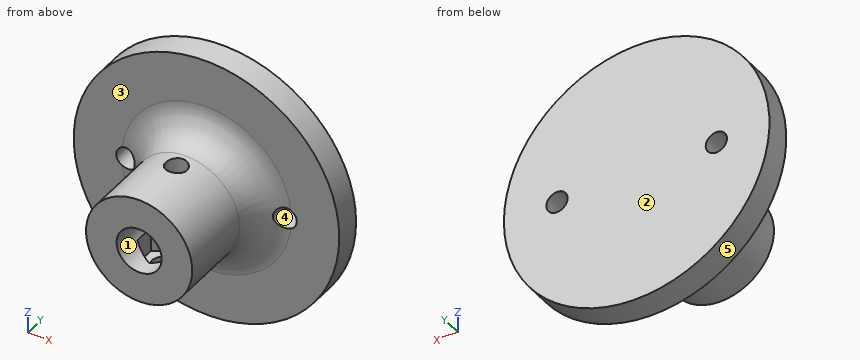
Solid Edge part; units mm, degrees
sketch "Sketch1" plane through (0, 0, 0) normal (0, -1, 0) x (1, 0, 0)
  circle A0 centre (0, 0) radius 10
  circle A1 centre (0, 0) radius 4.25
extrude "Protrusion1" add sketch "Sketch1" along normal blind 20
sketch "Sketch2" plane through (0, 0, 0) normal (0, -1, 0) x (1, 0, 0)
  circle A0 centre (-15, 0) radius 2
  circle A1 centre (0, 0) radius 25
  circle A2 centre (15, 0) radius 2
extrude "ExtrudedProtrusion_3" add sketch "Sketch2" against normal blind 5
fillet "Round_2" radius 6 1 edges at (-10, 0, 0)
sketch "Sketch3" plane through (0, 0, 0) normal (0, 0, 1) x (1, 0, 0)
  line L0 (-3.5, -10.9793) -> (-3.5, -15.0207)
  line L1 (-3.5, -15.0207) -> (0, -17.0415)
  line L2 (0, -17.0415) -> (3.5, -15.0207)
  line L3 (3.5, -15.0207) -> (3.5, -10.9793)
  line L4 (3.5, -10.9793) -> (0, -8.9585)
  line L5 (0, -8.9585) -> (-3.5, -10.9793)
extrude "ExtrudedCutout_3" cut sketch "Sketch3" against normal blind 7
sketch "Sketch4" plane through (0, 0, 0) normal (0, 0, 1) x (1, 0, 0)
  line L0 (0, -13) -> (3.5, -10.9793)
  line L1 (3.5, -10.9793) -> (3.5, -6.9378)
  line L2 (3.5, -6.9378) -> (0, -4.9171)
  line L3 (0, -4.9171) -> (-3.5, -6.9378)
  line L4 (-3.5, -6.9378) -> (-3.5, -10.9793)
  line L5 (-3.5, -10.9793) -> (0, -13)
extrude "ExtrudedCutout_4" cut sketch "Sketch4" along normal blind 7
sketch "Sketch5" plane through (0, 0, -11) normal (0, 0, 1) x (1, 0, 0)
  circle A0 centre (0, -13) radius 2
extrude "ExtrudedCutout_5" cut sketch "Sketch5" along normal blind 8
sketch "Sketch6" plane through (0, 0, 11) normal (0, 0, 1) x (1, 0, 0)
  circle A0 centre (0, -8.9585) radius 2
extrude "ExtrudedCutout_6" cut sketch "Sketch6" against normal blind 8
Source: CAD feature listing. Evaluate the final solid. Frame: model axes, mm. Face numbers are marked on the shaded views. A direction names the side the tool comes from. Round coordinates to 2 decimals unless told otherwise and drop trailing zeros. Loops run counter-clockwise (first coordinate to the right, second up) from the corner with the lowest first, then second, coordinate; pieces in that order, holes last. Notation, with made-up numbers: M -2.75,80.5 L 3.25,80.5 A8 ccw 3.25,85.5 Z; hole C 50.5,80.5 d1. An arc over 180 degrees is marked long. Use a Markdown table: item, result. Add a question column.
1. Line query: line 1 (X direction, y = -13, z = -9.05); line 2 (Z direction, x = 0, y = -16); line 3 (Z direction, x = 0, y = -10.5). Output: solid intervals per line, ascending.
2. Section query A-A on z = 0. Return the cut outline in (x, y).
3. Reachability of the marked faces 1 and 2 from +Z, -Z, +X, -X, +Y, -Y: full face, straight path, thin tool, end or side. Return the list, or none.
4. Section query B-B on y = 3.25. Return the cut outline in (x, z).
5. Section query D-D on z = 18. Return the cut outline in (x, y), then the cut area to 3 significant figures.
6. Contact query for flat-ended pins moving along their axis: P1, Ø4.5, axis at y = -13.5, z = -5.5, coming from the +X side; P2, Ø2, axis at x = 1.5, y = -9.5, coming from the -Z side; P3, Ø2.5, axis at x = 15, z = 0, coming from the -Y side; P4, Ø7.5, axis at x = 0.5, y = -11.5, coming from the +Z side. Output: stop coordinate, or through.
7. Section query C-C on y = -2.25. Return the cut outline in (x, z), then the cut area to 3 significant figures.
8. Mould query, pull axis X, two halves, no side actions, for the marked faces 3, 4 and 5. Classes: pulls with the +X half, pulls with the -X half, needs draft (parallel to the pull), parting line crosses it, or undercut.
Reported:
| question | item | result |
|---|---|---|
| 1 | line 1 | x = -4.25 to -2, 2 to 4.25 |
| 1 | line 2 | z = -10 to -7, 4.25 to 10 |
| 1 | line 3 | z = -10 to -7 |
| 2 | outline | M -25,0 L -17,0 L -17,5 L -25,5 Z; M -13,-0.8 A6 cw -10,-6 L -10,-20 L -4.25,-20 L -4.25,0 L 4.25,0 L 4.25,-20 L 10,-20 L 10,-6 A6 cw 13,-0.8 L 13,5 L -13,5 Z; M 17,0 L 25,0 L 25,5 L 17,5 Z |
| 3 | face 1 | -Y |
| 3 | face 2 | +Z, -Z, +X, -X, +Y |
| 4 | outline | C 0,0 d50; hole C -15,0 d4; hole C 15,0 d4 |
| 5 | outline | M -17.35,0 L 17.35,0 L 17.35,5 L -17.35,5 Z |
| 5 | area | 173 mm² |
| 6 | P1 | stops at x = 9.46 |
| 6 | P2 | stops at z = -9.99 |
| 6 | P3 | passes through |
| 6 | P4 | stops at z = 10 |
| 7 | outline | C 0,0 d22.63; hole C 0,0 d8.5 |
| 7 | area | 346 mm² |
| 8 | face 3 | needs draft |
| 8 | face 4 | undercut |
| 8 | face 5 | parting line crosses it |
